Part model, mm, in its own coordinate system. A direction names the side the tool comes from. Round coordinates to 2 decimals unless told otherwise and drop trailing zeros. Write each loop counter-clockwise with the first axis right and the second up, starting at its lowest first coordinate (ties: lowest second). Pieces come first, ordered by that corner, then holes. Notation, with made-up numbers: (-9.75, 61) -> (-2.75, 61) arc R28 ccw to (-2.75, 84) -> close; hole circle Ø3 at (-20, 8). An arc over 180 degrees is marked (long way). Return JSON: item names as keys, results as strings. Group by question number.
```python
from build123d import *

# Parameters (mm, degrees)
TOP_ENCLOSURE_DEPTH    = 77
TOP_EXTRA_DEPTH        = 12
SKETCH3_W              = 35
SKETCH3_H              = 42
SOLAR_CELL_SLOT_DEPTH  = 2
SKETCH4_R              = 1.5
SOLAR_CELL_HOLES_DEPTH = 108.30330843
BOSS_EXTRUDE1_REACH    = 108.922
BOSS_EXTRUDE2_REACH    = 120.819
FILLET1_R              = 7.5


with BuildPart() as part:
    # Master_Geometry → Top_Enclosure (new body)
    with BuildSketch(Plane.XY):
        Polygon((-48, -3.5), (-53, -3.5), (-42.080892972, 26.5), (42.080892972, 26.5), (53, -3.5), (48, -3.5), (48, 4), (38, 4), (38, 21.5), (-38, 21.5), (-38, 4), (-48, 4), align=None)
    extrude(amount=TOP_ENCLOSURE_DEPTH)

    # Sketch2 → Top_Extra (add)
    with BuildSketch(Plane.XY.offset(77)):
        Polygon((-42.080892972, 26.5), (42.080892972, 26.5), (53, -3.5), (-53, -3.5), align=None)
    top_extra = extrude(amount=TOP_EXTRA_DEPTH)

    # Mirror1: Top_Extra across plane
    add(top_extra.mirror(Plane(origin=(0, 0, 38.5), x_dir=(1, 0, 0), z_dir=(0, 0, -1))))

    # Sketch3 → Solar_Cell_Slot (cut)
    with BuildSketch(Plane(origin=(0, 26.5, 0), x_dir=(1, 0, 0), z_dir=(0, 1, 0))):
        with Locations((14.580892972, -38.5)):
            Rectangle(SKETCH3_W, SKETCH3_H)
    extrude(amount=-SOLAR_CELL_SLOT_DEPTH, mode=Mode.SUBTRACT)

    # Sketch4 → Solar_Cell_Holes (cut, through all)
    with BuildSketch(Plane(origin=(0, 24.5, 0), x_dir=(1, 0, 0), z_dir=(0, 1, 0))):
        with Locations(Location((1.330892972, -34.125, 0), (0, 0, 270))):
            Circle(SKETCH4_R)
        with Locations(Location((1.330892972, -42.875, 0), (0, 0, 270))):
            Circle(SKETCH4_R)
    extrude(amount=-SOLAR_CELL_HOLES_DEPTH, mode=Mode.SUBTRACT)

    # Boss-Extrude1: up to this plane
    boss_extrude1_end = Plane(origin=(42.080892972, 26.5, 77), z_dir=(-0.9396926207859069, -0.3420201433256729, 0))
    # Sketch5 → Boss-Extrude1 (add, up to the surface)
    with BuildSketch(Plane(origin=(0, 0, 0), x_dir=(0, 0, -1), z_dir=(1, 0, 0)), mode=Mode.PRIVATE) as boss_extrude1_sk1:
        Polygon((-89, 26.5), (-89, -3.5), (-102.989229745, -3.5), align=None)
    boss_extrude1_tool1 = split(extrude(boss_extrude1_sk1.sketch, amount=BOSS_EXTRUDE1_REACH, mode=Mode.PRIVATE), bisect_by=boss_extrude1_end, keep=Keep.BOTH, mode=Mode.PRIVATE)
    boss_extrude1 = boss_extrude1_tool1.solids().sort_by_distance((0, 6.5, 93.663077))[0]
    add(boss_extrude1)

    # Boss-Extrude2: up to this face of the body (flat: up to its plane)
    boss_extrude2_end = Plane(part.part.faces().sort_by_distance((-47.540446486, 11.5, 38.5))[0])
    # Sketch6 → Boss-Extrude2 (add, up to the picked face)
    with BuildSketch(Plane.ZY, mode=Mode.PRIVATE) as boss_extrude2_sk1:
        Polygon((89, 26.5), (102.989229745, -3.5), (89, -3.5), align=None)
    boss_extrude2_tool1 = split(extrude(boss_extrude2_sk1.sketch, amount=BOSS_EXTRUDE2_REACH, mode=Mode.PRIVATE), bisect_by=boss_extrude2_end, keep=Keep.BOTH, mode=Mode.PRIVATE)
    boss_extrude2 = boss_extrude2_tool1.solids().sort_by(Axis((0, 6.5, 93.663077), (-1, 0, 0)))[0]
    add(boss_extrude2)

    # Mirror3: Boss-Extrude1, Boss-Extrude2 across plane
    add(boss_extrude1.mirror(Plane(origin=(0, 0, 38.5), x_dir=(1, 0, 0), z_dir=(0, 0, -1))))
    add(boss_extrude2.mirror(Plane(origin=(0, 0, 38.5), x_dir=(1, 0, 0), z_dir=(0, 0, -1))))

    # Fillet1
    fillet1_edges = [part.edges().sort_by_distance(p)[0] for p in [
        (-47.540446486, 11.5, 95.994614872),
        (47.540446486, 11.5, -18.994614872),
        (-47.540446486, 11.5, -18.994614872),
        (47.540446486, 11.5, 95.994614872),
    ]]
    fillet(fillet1_edges, radius=FILLET1_R)


solid = part.part
```
Item 1: Cut at B-B (x = 26.5). Write the cut outline in (y, z), then the cut area to 3 significant figures.
Item 2: Wall check: L1, parallel to Y at x = 37.5, z = 19; L2, parallel to Z at x = -38, y = 0; L3, parallel to Z at x = -5, y = 6. Give the ranges that are in metal, low to high.
Item 3: Which spindle directions (+Z, -Z, +X, -X, +Y, -Y) get a long thin tool onto all of the face, cutting with end or side? Do faces 4 (the face through (1.397, 23.021, 41.376)), 5 (the face through (38, 13, 38)), 6 (the face through (14, 24.5, 38)). Say none if no direction does.
Item 4: Two-plate mould, pull along Z, no slides. Class faces 1 (the face through (0.6, 11.7, -18.9)), 2 (the face through (1, 9, 77)), 3 (the face through (-10, 26.5, 39)): released by +Z, released by -Z, zero draft, split by the parting line, or undercut.
Item 5: Cut at C-C (z = 29.5). Write the cut outline in (x, y).
Item 6: Cut at D-D (x = -21). Write the cut outline in (y, z), then the cut area to 3 significant figures.
Item 7: Cut at A-A (z = 8.5). Write the cut outline in (x, y).
Item 8: Flat gauge pins, fed straight in: P1, Ø5, axis at y = 10.5, z = 27, coming from the -X side; P2, Ø3, axis at y = 18.5, z = 19.5, coming from the -X side; P3, Ø8, axis at y = 1, z = 49, coming from the -X side; P4, Ø11, axis at x = 43, z = 41.5, coming from the -Y side. Where does each tip first touch, or does it go through?
Checks:
{
 "1": {"outline": "(-3.5, -25.99) -> (26.5, -12) -> (26.5, 17.5) -> (24.5, 17.5) -> (24.5, 59.5) -> (26.5, 59.5) -> (26.5, 89) -> (-3.5, 102.99) -> (-3.5, 77) -> (21.5, 77) -> (21.5, 0) -> (-3.5, 0) -> close", "area": "1,440 mm2"},
 "2": {"L1": "y = 21.5 to 26.5", "L2": "z = -24.36 to 0, 77 to 101.36", "L3": "z = -21.56 to 0, 77 to 98.56"},
 "3": {"face 4": "+Y, -Y", "face 5": "-Y", "face 6": "+Y"},
 "4": {"face 1": "released by -Z", "face 2": "undercut", "face 3": "zero draft"},
 "5": {"outline": "(-53, -3.5) -> (-48, -3.5) -> (-48, 4) -> (-38, 4) -> (-38, 21.5) -> (38, 21.5) -> (38, 4) -> (48, 4) -> (48, -3.5) -> (53, -3.5) -> (42.08, 26.5) -> (32.08, 26.5) -> (32.08, 24.5) -> (-2.92, 24.5) -> (-2.92, 26.5) -> (-42.08, 26.5) -> close"},
 "6": {"outline": "(-3.5, -25.99) -> (26.5, -12) -> (26.5, 89) -> (-3.5, 102.99) -> (-3.5, 77) -> (21.5, 77) -> (21.5, 0) -> (-3.5, 0) -> close", "area": "1,520 mm2"},
 "7": {"outline": "(-53, -3.5) -> (-48, -3.5) -> (-48, 4) -> (-38, 4) -> (-38, 21.5) -> (38, 21.5) -> (38, 4) -> (48, 4) -> (48, -3.5) -> (53, -3.5) -> (42.08, 26.5) -> (-42.08, 26.5) -> close"},
 "8": {"P1": "stops at x = -48.81", "P2": "stops at x = -45.54", "P3": "stops at x = -52.82", "P4": "stops at y = -3.5"}
}
